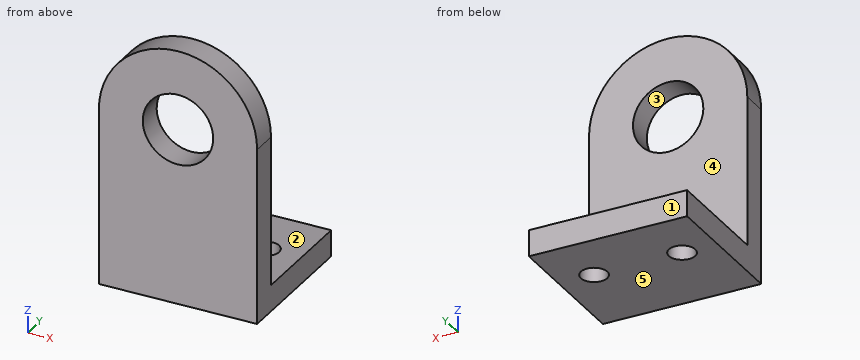
from build123d import *

# Parameters (mm, degrees)
SKETCH_1_W      = 18
SKETCH_1_H      = 16
SKETCH_1_R      = 1.5
EXTRUDE_1_DEPTH = 3
SKETCH_3_R      = 4
EXTRUDE_2_DEPTH = 3


with BuildPart() as part:
    # 草图1 → 凸台-拉伸1 (new body)
    with BuildSketch(Plane.XY):
        Rectangle(SKETCH_1_W, SKETCH_1_H)
        with Locations((-5, 1.5)):
            Circle(SKETCH_1_R, mode=Mode.SUBTRACT)
        with Locations(Location((5, 1.5, 0), (0, 0, 180))):
            Circle(SKETCH_1_R, mode=Mode.SUBTRACT)
    extrude(amount=EXTRUDE_1_DEPTH)

    # 草图3 → 凸台-拉伸2 (add)
    with BuildSketch(Plane.XZ.offset(8)):
        with BuildLine():
            Line((-9, 0), (9, 0))
            Line((9, 0), (9, 20))
            ThreePointArc((9, 20), (0, 29), (-9, 20))
            Line((-9, 20), (-9, 0))
        make_face()
        with Locations(Location((0, 20, 0), (0, 0, 270))):
            Circle(SKETCH_3_R, mode=Mode.SUBTRACT)
    extrude(amount=-EXTRUDE_2_DEPTH)


solid = part.part
Design review of the part built by this model. Coordinates are the model's own, in mm. Face numbers are marked on the shaded views. A direction names the side the tool comes from. Coordinates: 2 decimals unless noted, no trailing zeros. Loops run counter-clockwise (first coordinate to the right, second up) from the corner with the lowest first, then second, coordinate; pieces in that order, holes last. Notation, with made-up numbers: (-27.75, 64.5) -> (-5.75, 64.5) arc R26 cw to (-5.75, 97.5) -> close; hole circle Ø3 at (-29, -13.5). An arc over 180 degrees is marked (long way). Use a Markdown table: item, result. Add a question column.
Item 1: Machinability: for the marked faces 1 and 2, which of the approach directions +Z, -Z, +X, -X, +Y, -Y give a long, thin tool a straight path to every point of the face, cutting with its end or side? Answer none if there is none.
Item 2: We need section B-B, the plane y = 1.5. Write out the cut boundary in (x, z).
Item 3: We need section D-D, the plane z = 22. Write out the cut boundary in (x, y), and give its area (3 significant figures).
Item 4: The part is to be moulded in two halves that separate along Z. For the marked faces 3, 4 and 5, say which applies: +Z half, -Z half, draft (parallel to the pull), parting line (faces both ways), or undercut.
Item 5: Clearance check with flat-ended pins moving along their axes: P1, Ø4, axis at x = 3, y = 2, coming from the +Z side; P2, Ø5.5, axis at x = -3, z = 18, coming from the +Y side. State where each tip first meets the part, or that it passes through.
Item 6: We need section C-C, the plane y = -7. Write out the cut boundary in (x, z).
Item 7: We need section A-A, the plane x = 0. Write out the cut boundary in (y, z), and give its area (3 significant figures).
Item 8: Wall thickness on L1, parallel to Y at x = 5, z = 2.05; L2, parallel to Y at x = 3.25, z = 5.75; L3, parallel to Z at x = 2.5, y = -2.5: over which ranges is each line inside the solid? List them lowest first. Write a range as from..to.
Numbers:
| question | item | result |
|---|---|---|
| 1 | face 1 | +Z, -Z, +X, -X, +Y |
| 1 | face 2 | +Z, +X, -X, +Y |
| 2 | outline | (-9, 0) -> (-6.5, 0) -> (-6.5, 3) -> (-9, 3) -> close; (-3.5, 0) -> (3.5, 0) -> (3.5, 3) -> (-3.5, 3) -> close; (6.5, 0) -> (9, 0) -> (9, 3) -> (6.5, 3) -> close |
| 3 | outline | (-8.77, -8) -> (-3.46, -8) -> (-3.46, -5) -> (-8.77, -5) -> close; (3.46, -8) -> (8.77, -8) -> (8.77, -5) -> (3.46, -5) -> close |
| 3 | area | 31.9 mm^2 |
| 4 | face 3 | undercut |
| 4 | face 4 | draft |
| 4 | face 5 | -Z half |
| 5 | P1 | stops at z = 3 |
| 5 | P2 | stops at y = -5 |
| 6 | outline | (-9, 0) -> (9, 0) -> (9, 20) arc R9 ccw to (-9, 20) -> close; hole circle Ø8 at (0, 20) |
| 7 | outline | (-8, 0) -> (8, 0) -> (8, 3) -> (-5, 3) -> (-5, 16) -> (-8, 16) -> close; (-8, 24) -> (-5, 24) -> (-5, 29) -> (-8, 29) -> close |
| 7 | area | 102 mm^2 |
| 8 | L1 | y = -8..0, 3..8 |
| 8 | L2 | y = -8..-5 |
| 8 | L3 | z = 0..3 |
